Source: three-view drawing plus pictorial views. Frame: mm from the lowest corner of the part. Give positions to 0.01 mm unless a question says otherwise; leave off trailing zeros. Loops run counter-clockwise (first coordinate to the right, second up) from the corner with the lowest first, then second, coordinate; pieces in that order, holes last. Notation, with made-up numbers: (13.25, 22.25) -> (61.25, 22.25) arc R12 cw to (61.25, 30.25) -> close; hole circle Ø6 at (69, 33). An arc over 180 degrees is marked (long way). Answer as a JSON object with one key per item and string values. Group by question number.
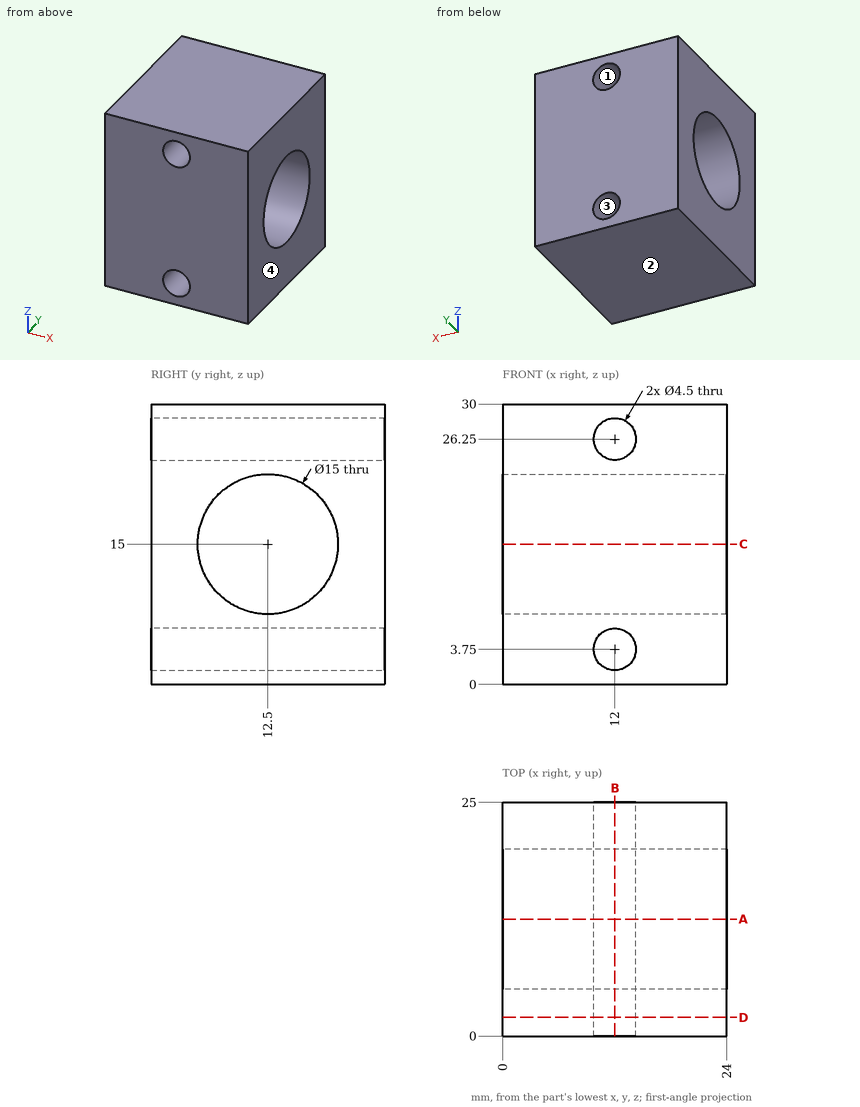
Q1. Ray query, probe 1 along Y at (x, z) = (9.75, 15); probe 2 along X at (y, z) = (8.75, 3.75); probe 3 along Z at (x, y) = (11.25, 12.25). Return the intervals inside material, ascending.
Q2. Pin query (flat end, axial travel): pin 1 Ø1 at (x, y) = (17.5, 12.5) entering from -Z; pin 2 Ø13.5 at (y, z) = (12.5, 15) entering from -X. Return the tip coordinate at first contact, or that it passes through.
Q3. Section C-C on z = 15. Return the cut outline in (x, y), then the cut area to 3 significant figures.
Q4. Section D-D on y = 2. Return the cut outline in (x, z), then the cut area to 3 significant figures.
Q5. Section A-A on y = 12.5. Return the cut outline in (x, z).
Q6. Section B-B on x = 12. Return the cut outline in (y, z), then the cut area to 3 significant figures.
Q7. Pull-direction query (X, two-part tool) for the marked faces 1, 2, 3 and 4; classes: +X half, -X half, draft (parallel to the pull), parting line (faces both ways), or undercut.
Numbers:
{
 "1": {"probe 1": "y = 0 to 5, 20 to 25", "probe 2": "x = 0 to 9.75, 14.25 to 24", "probe 3": "z = 0 to 1.63, 5.87 to 7.5, 22.5 to 24.13, 28.37 to 30"},
 "2": {"pin 1": "stops at z = 0", "pin 2": "passes through"},
 "3": {"outline": "(0, 0) -> (24, 0) -> (24, 5) -> (0, 5) -> close; (0, 20) -> (24, 20) -> (24, 25) -> (0, 25) -> close", "area": "240 mm²"},
 "4": {"outline": "(0, 0) -> (24, 0) -> (24, 30) -> (0, 30) -> close; hole circle Ø4.5 at (12, 3.75); hole circle Ø4.5 at (12, 26.25)", "area": "688 mm²"},
 "5": {"outline": "(0, 0) -> (24, 0) -> (24, 7.5) -> (0, 7.5) -> close; (0, 22.5) -> (24, 22.5) -> (24, 30) -> (0, 30) -> close; hole circle Ø4.5 at (12, 3.75); hole circle Ø4.5 at (12, 26.25)"},
 "6": {"outline": "(0, 0) -> (25, 0) -> (25, 1.5) -> (0, 1.5) -> close; (0, 6) -> (25, 6) -> (25, 24) -> (0, 24) -> close; (0, 28.5) -> (25, 28.5) -> (25, 30) -> (0, 30) -> close; hole circle Ø15 at (12.5, 15)", "area": "348 mm²"},
 "7": {"face 1": "undercut", "face 2": "draft", "face 3": "undercut", "face 4": "+X half"}
}
